from build123d import *

# Parameters (mm, degrees)
F0_W     = 86.8310853839
F0_H     = 83.1971988082
F1_DEPTH = 13.208
F2_R     = 0.508
F3_T     = 0.508
F4_W     = 63.2273703814
F4_H     = 62.8109127283
F5_DEPTH = 17.272


# Not quite as in the source:
# - a shell that OpenCascade refuses in one call is made with other operations: the cavity is built on its own and cut out


with BuildPart() as f1:
    # F0 (on Top) → F1 (new body)
    with BuildSketch(Plane.XY):
        Rectangle(F0_W, F0_H)
    extrude(amount=F1_DEPTH)

    # F2
    f2_edges = [f1.edges().sort_by_distance(p)[0] for p in [
        (0, -41.598599, 13.208),
        (-43.415543, 0, 13.208),
        (0, 41.598599, 13.208),
        (43.415543, 0, 13.208),
    ]]
    fillet(f2_edges, radius=F2_R)

    # F3: shell of thickness 0.508, made by hand


with BuildPart() as f3_core1:
    # F3_t2: copy of F1
    add(f1.part)

    # the walls: a layer under each face that stays
    f3_faces = [f3_core1.faces().sort_by_distance(p)[0] for p in [
        (0, -41.5985994041, 6.35),
        (-43.4155426919, 0, 6.35),
        (43.4155426919, 0, 6.35),
        (0, 41.5985994041, 6.35),
        (0, 0, 13.208),
    ]]
    thicken(f3_faces, amount=-F3_T, mode=Mode.SUBTRACT)


with BuildPart() as f1_1:
    add(f1.part)

    # what is left inside the walls is the cavity
    f3_cavity = [f3_core1.part.solids().sort_by_distance(p)[0] for p in [
        (0, -13.696866, 12.69492),
    ]]
    add(f3_cavity, mode=Mode.SUBTRACT)

    # F4 (on face) → F5 (cut)
    with BuildSketch(Plane.XY.offset(13.208)):
        Rectangle(F4_W, F4_H)
    extrude(amount=-F5_DEPTH, mode=Mode.SUBTRACT)


solid = f1_1.part
Geometry check sheet. Reference: the model listing, model coordinates, mm. A direction names the side the tool comes from. Give positions to 0.01 mm unless a question says otherwise; leave off trailing zeros. Order: outer loops, then holes, each group sorted by start corner. A loop starts at its lowest first (then second) coordinate and runs counter-clockwise, first axis right, second up.
1. Scan lines: line 1 (Y direction, x = -38.5, z = 3.75); line 2 (X direction, y = 25, z = 4.25); line 3 (Z direction, x = 19, y = -33.5). Record each from-to range of solid material in increasing order.
Completed:
line 1: y = -41.6 to -41.09, 41.09 to 41.6
line 2: x = -43.42 to -42.91, 42.91 to 43.42
line 3: z = 12.7 to 13.21
2. Sectioned sample at D-D (x = 37). Record the boundary of the cut face in (y, z), then the cut area to 3 significant figures.
Completed:
outline: (-41.6, 0) - (-41.09, 0) - (-41.09, 12.7) - (41.09, 12.7) - (41.09, 0) - (41.6, 0) - (41.6, 12.7) arc R0.51 ccw to (41.09, 13.21) - (-41.09, 13.21) arc R0.51 ccw to (-41.6, 12.7) - close
area: 55.1 mm2
3. Draft check along Y on faces 1 (the face through (-42.908, -1, 6)), 2 (the face through (43.416, -1, 6)), 3 (the face through (-1, 41.091, 6)), 4 (the face through (-1, -41.599, 6)). Enter one of: pulls with the +Y half, pulls with the -Y half, needs draft (parallel to the pull), parting line crosses it, or undercut.
Completed:
face 1: undercut
face 2: needs draft
face 3: undercut
face 4: pulls with the -Y half
4. Sectioned sample at C-C (z = 8). Record the boundary of the cut face in (x, y).
Completed:
outline: (-43.42, -41.6) - (43.42, -41.6) - (43.42, 41.6) - (-43.42, 41.6) - close; hole (-42.91, -41.09) - (42.91, -41.09) - (42.91, 41.09) - (-42.91, 41.09) - close
5. Sectioned sample at A-A (y = 28). Record the boundary of the cut face in (x, z), then the cut area to 3 significant figures.
Completed:
outline: (-43.42, 0) - (-42.91, 0) - (-42.91, 12.7) - (-31.61, 12.7) - (-31.61, 13.21) - (-42.91, 13.21) arc R0.51 ccw to (-43.42, 12.7) - close; (31.61, 12.7) - (42.91, 12.7) - (42.91, 0) - (43.42, 0) - (43.42, 12.7) arc R0.51 ccw to (42.91, 13.21) - (31.61, 13.21) - close
area: 24.8 mm2
6. Access from +Z, -Z, +X, -X, +Y, -Y to the whole of each face (thin tool, end or side, straight path). Record for faces 5 (the face through (-1, -36, 13.208)), 6 (the face through (42.908, -1, 6)).
Completed:
face 5: +Z, +X, -X, +Y, -Y
face 6: -Z
7. Sectioned sample at B-B (x = 18). Record the boundary of the cut face in (y, z).
Completed:
outline: (-41.6, 0) - (-41.09, 0) - (-41.09, 12.7) - (-31.41, 12.7) - (-31.41, 13.21) - (-41.09, 13.21) arc R0.51 ccw to (-41.6, 12.7) - close; (31.41, 12.7) - (41.09, 12.7) - (41.09, 0) - (41.6, 0) - (41.6, 12.7) arc R0.51 ccw to (41.09, 13.21) - (31.41, 13.21) - close
